Could you check a few things on this model? Use its own coordinates, in mm. Face numbers are marked on the shaded views. A direction names the side the tool comes from. Round coordinates to 2 decimals unless told otherwise and drop trailing zeros. Write each loop counter-clockwise with the first axis right and the second up, starting at its lowest first coordinate (ties: lowest second). Pieces come first, ordered by that corner, then holes. Notation, with made-up numbers: (21, -26) -> (57, -26) arc R34 ccw to (57, 5) -> close; hole circle Ø7 at (52, 3.5). An arc over 180 degrees is marked (long way). One line per question, with ' | ' between items. Start each with the question number.
1. Imagine slicing it at D-D, the plane x = 146.25. List the corners of the cut face in (y, z) for me.
2. If I drill on line 1 along X through (y, z) = (-11.5, 9.5); line 2 along Y through (x, z) = (150, 22.5); line 3 along Y through (x, z) = (156, 27.5), over which ranges is the centre line in solid material (lowest first)? Write a range as [from, to].
3. Thinking about a two-plate mould opening in Z: for the marked faces 1, 2 and 3, which applies, released by +Z, released by -Z, zero draft, split by the parting line, or undercut?
4. For the marked faces 4, 5, 6 and 7, which set-ups out of +Z, -Z, +X, -X, +Y, -Y let a thin tool reach every point of the face, with its end or its side?
5. Imagine slicing it at C-C, the plane y = -60.5. List the corners of the cut face in (x, z) for me.
6. Imagine slicing it at A-A, the plane y = -85. List the corners of the cut face in (x, z) for me, and give its area (3 significant figures).
7. For pin 1 Ø3 at (x, y) = (133.5, -43) entering from +Z; pin 2 Ø2 at (x, z) = (143, 19) entering from -Y; pin 3 Ø3 at (x, y) = (152, 20.5) entering from +Z, each with a flat end and sliding along its axis, tell me the tip position at first contact or that it passes through.
8. Imagine slicing it at B-B, the plane x = 140. List the corners of the cut face in (y, z) for me, and give its area (3 significant figures).
from build123d import *

# Parameters (mm, degrees)
F1_DEPTH     = 22
F2_W         = 30
F2_H         = 135
F3_DEPTH     = 2
F4_W         = 30
F4_H         = 25.5063175828
F4_R         = 2.5
F5_DEPTH     = 10
F6_W         = 30
F6_H         = 10
F7_DEPTH     = 3
F8_T1_DEPTH  = 4
F8_T3_DEPTH  = 4
F8_T8_DEPTH  = 4
F8_T13_DEPTH = 4


# Not quite as in the source:
# - a fillet or chamfer that OpenCascade refuses, or shapes differently, is made with other operations: its cross-section is extruded or revolved along the edge and cut away or added


with BuildPart() as f1:
    # F0 (on Top) → F1 (new body)
    with BuildSketch(Plane.XY):
        Polygon((160.7300297916, 27.1383413836), (130.7300297916, 27.1383413836), (130.7300297916, -107.8616586164), (134.7300297916, -107.8616586164), (134.7300297916, -105.3616586164), (134.7300297916, 24.6383413836), (156.7300297916, 24.6383413836), (156.7300297916, -105.3616586164), (156.7300297916, -107.8616586164), (160.7300297916, -107.8616586164), align=None)
    extrude(amount=F1_DEPTH)

    # F2 (on face) → F3 (join)
    with BuildSketch(Plane(origin=(0, 0, 0), x_dir=(1, 0, 0), z_dir=(0, 0, -1))):
        with Locations((145.7300297916, 40.3616586164)):
            Rectangle(F2_W, F2_H)
    extrude(amount=F3_DEPTH)

    # F4 (on face) → F5 (join)
    with BuildSketch(Plane.XY.offset(22)):
        with Locations((145.7300297916, -90.3616586164)):
            Rectangle(F4_W, F4_H)
        with Locations((145.7300297916, -90.3616586164)):
            Circle(F4_R, mode=Mode.SUBTRACT)
    extrude(amount=F5_DEPTH)

    # F6 (on face) → F7 (join)
    with BuildSketch(Plane.XY.offset(22)):
        with Locations((145.7300297916, 22.1383413836)):
            Rectangle(F6_W, F6_H)
    extrude(amount=F7_DEPTH)

    # F8: chamfer of 5 on 4 edges, made by hand

    # F8_s2 → F8_t1 (join)
    with BuildSketch(Plane.YZ.offset(156.7300297916)):
        Polygon((-72.608499825, 22), (-77.608499825, 27), (-77.608499825, 22), align=None)
    extrude(amount=F8_T1_DEPTH)

    # F8_s4 → F8_t3 (join)
    with BuildSketch(Plane.YZ.offset(130.7300297916)):
        Polygon((-77.608499825, 27), (-72.608499825, 22), (-77.608499825, 22), align=None)
    extrude(amount=F8_T3_DEPTH)


with BuildPart() as f8_tool6:
    # F8_s7 → F8_t8 (new body)
    with BuildSketch(Plane.YZ.offset(130.7300297916)):
        Polygon((-103.1148174078, 27), (-108.1148174078, 22), (-103.1148174078, 22), align=None)
    extrude(amount=F8_T8_DEPTH)

    split(bisect_by=Plane.XZ.offset(107.8616586164), keep=Keep.BOTTOM)


with BuildPart() as f1_1:
    add(f1.part)

    # F8_t5: union F8_tool6
    add(f8_tool6.part)


with BuildPart() as f8_tool11:
    # F8_s12 → F8_t13 (new body)
    with BuildSketch(Plane.YZ.offset(156.7300297916)):
        Polygon((-103.1148174078, 27), (-108.1148174078, 22), (-103.1148174078, 22), align=None)
    extrude(amount=F8_T13_DEPTH)

    split(bisect_by=Plane.XZ.offset(107.8616586164), keep=Keep.BOTTOM)


with BuildPart() as f1_2:
    add(f1_1.part)

    # F8_t10: union F8_tool11
    add(f8_tool11.part)


solid = f1_2.part
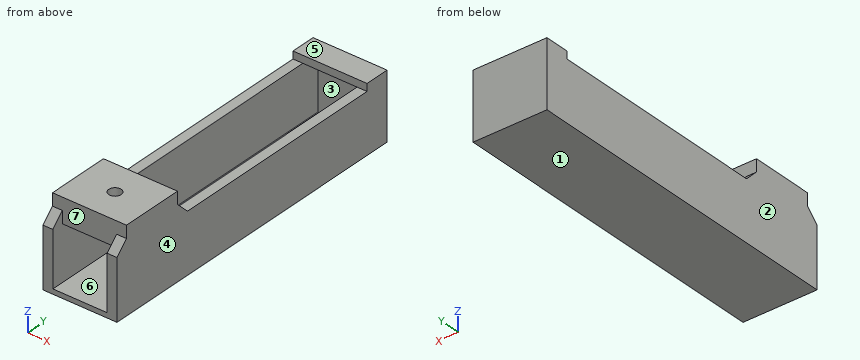
Geometry results:
1) outline: (-107.86, -2) -> (27.14, -2) -> (27.14, 25) -> (17.14, 25) -> (17.14, 22) -> (24.64, 22) -> (24.64, 0) -> (-107.86, 0) -> close; (-103.11, 22) -> (-92.81, 22) -> (-92.81, 32) -> (-103.11, 32) -> close; (-87.92, 22) -> (-77.61, 22) -> (-77.61, 32) -> (-87.92, 32) -> close
2) line 1: x = [130.73, 134.73], [156.73, 160.73] | line 2: y = [-103.11, -77.61], [17.14, 27.14] | line 3: y = [-103.11, -77.61]
3) face 1: released by -Z | face 2: zero draft | face 3: undercut
4) face 4: +Z, -Z, +X, +Y, -Y | face 5: +Z, +X, -X, +Y | face 6: -Y | face 7: +Z, -Y
5) outline: (130.73, -2) -> (160.73, -2) -> (160.73, 22) -> (156.73, 22) -> (156.73, 0) -> (134.73, 0) -> (134.73, 22) -> (130.73, 22) -> close
6) outline: (130.73, -2) -> (160.73, -2) -> (160.73, 32) -> (130.73, 32) -> close; hole (134.73, 0) -> (156.73, 0) -> (156.73, 22) -> (134.73, 22) -> close | area: 536 mm2
7) pin 1: stops at z = 22 | pin 2: stops at y = 24.64 | pin 3: stops at z = 25
8) outline: (-107.86, -2) -> (27.14, -2) -> (27.14, 25) -> (17.14, 25) -> (17.14, 22) -> (24.64, 22) -> (24.64, 0) -> (-107.86, 0) -> close; (-103.11, 22) -> (-77.61, 22) -> (-77.61, 32) -> (-103.11, 32) -> close | area: 610 mm2
